from build123d import *

# Parameters (mm, degrees)
BOSS_EXTRUDE1_DEPTH = 15.7
LPATTERN1_COUNT     = 8
LPATTERN1_PITCH     = 8
SKETCH2_W           = 1.2
SKETCH2_H           = 6.1
CUT_EXTRUDE1_DEPTH  = 67.562602113
SKETCH3_W           = 0.8
SKETCH3_H           = 3.2
BOSS_EXTRUDE2_DEPTH = 15.7


with BuildPart() as part:
    # Sketch1 → Boss-Extrude1 (new body)
    with BuildSketch(Plane(origin=(0, 0, 0), x_dir=(1, 0, 0), z_dir=(0, 1, 0))):
        with BuildLine():
            Line((0, 10.8), (0, 15.5))
            Line((0, 15.5), (5.6, 15.5))
            Line((5.6, 15.5), (5.6, 10.8))
            Line((5.6, 10.8), (6.8, 10.8))
            Line((6.8, 10.8), (6.8, 9.75))
            ThreePointArc((6.8, 9.75), (4.8, 7.75), (6.8, 5.75))
            Line((6.8, 5.75), (6.8, 4.7))
            Line((6.8, 4.7), (5.6, 4.7))
            Line((5.6, 4.7), (5.6, 0))
            Line((5.6, 0), (0, 0))
            Line((0, 0), (0, 4.7))
            Line((0, 4.7), (-1.2, 4.7))
            Line((-1.2, 4.7), (-1.2, 5.75))
            ThreePointArc((-1.2, 5.75), (0.8, 7.75), (-1.2, 9.75))
            Line((-1.2, 9.75), (-1.2, 10.8))
            Line((-1.2, 10.8), (0, 10.8))
        make_face()
    boss_extrude1 = extrude(amount=BOSS_EXTRUDE1_DEPTH)

    # LPattern1: Boss-Extrude1 ×8
    with Locations(*[(i * LPATTERN1_PITCH, 0, 0) for i in range(1, LPATTERN1_COUNT)]):
        add(boss_extrude1)

    # Sketch2 → Cut-Extrude1 (cut, through all)
    with BuildSketch(Plane(origin=(0, 15.7, 0), x_dir=(1, 0, 0), z_dir=(0, 1, 0))):
        with Locations((-0.6, 7.75)):
            Rectangle(SKETCH2_W, SKETCH2_H)
        with Locations((62.2, 7.75)):
            Rectangle(SKETCH2_W, SKETCH2_H)
    extrude(amount=-CUT_EXTRUDE1_DEPTH, mode=Mode.SUBTRACT)

    # Sketch3 → Boss-Extrude2 (add)
    with BuildSketch(Plane(origin=(0, 15.7, 0), x_dir=(1, 0, 0), z_dir=(0, 1, 0))):
        with Locations((0.4, 7.75)):
            Rectangle(SKETCH3_W, SKETCH3_H)
        with Locations((61.2, 7.75)):
            Rectangle(SKETCH3_W, SKETCH3_H)
    extrude(amount=-BOSS_EXTRUDE2_DEPTH)


solid = part.part
Work out the finished part from the listing and answer in its coordinate system (mm). A direction names the side the tool comes from. Give positions to 0.01 mm unless a question says otherwise; leave off trailing zeros. Order: outer loops, then holes, each group sorted by start corner. A loop starts at its lowest first (then second) coordinate and runs counter-clockwise, first axis right, second up. Notation, with made-up numbers: (0, -35.5) -> (33, -35.5) arc R23 ccw to (33, -0.5) -> close; hole circle Ø7 at (65.5, 85.25). An arc over 180 degrees is marked (long way). Answer as a JSON object with one key per item and string values. Group by question number.
1. Flat-ended cylindrical pins translate along their axes: pin 1 Ø3.5 at (x, z) = (6.8, -7.75) entering from +Y; pin 2 Ø1.9 at (x, y) = (55, 5) entering from -Z. Find the tip coordinate at first contact, or state that the pin passes through.
2. Section A-A on x = 22.8 is taken. Determine the outline of the cut face in (y, z), plus the area to 3 significant figures.
3. A tool of negligible diameter and unlimited length cuts with its end or side. For faces 1 (the flat face through (47, 8, -10.8)), 2 (the flat face through (45.6, 8, -2)), 3 (the flat face through (51, 8, 0)), from which of +Z, -Z, +X, -X, +Y, -Y can it reach the whole face along a straight path? Write none if from no direction.
4. Consider line 1 along Z through (x, y) = (38.8, 11); line 2 along Z through (x, y) = (29.5, 14). Determine where each line is inside the solid, lowest interval first. Write a range as [from, to].
5. The mould has two halves that part along Z. Classify faces 4 (the flat face through (37.6, 8, -2)), 5 (the flat face through (23, 8, -4.7)), 6 (the flat face through (51, 8, -15.5)), 7 (the cylindrical face through (30.712, 7.74, -5.752)): released by +Z, released by -Z, zero draft, split by the parting line, or undercut.
6. Section B-B on z = -4 is taken. Count the separate pieces of the cut face and the enclosed holes in it, plus the area to 3 significant figures.
Result sheet:
{
 "1": {"pin 1": "passes through", "pin 2": "stops at z = -10.8"},
 "2": {"outline": "(0, -10.8) -> (15.7, -10.8) -> (15.7, -9.75) -> (0, -9.75) -> close; (0, -5.75) -> (15.7, -5.75) -> (15.7, -4.7) -> (0, -4.7) -> close", "area": "33.0 mm^2"},
 "3": {"face 1": "-Z, +Y, -Y", "face 2": "+Z, +Y, -Y", "face 3": "+Z, +X, -X, +Y, -Y"},
 "4": {"line 1": "z = [-10.8, -9.75], [-5.75, -4.7]", "line 2": "z = [-15.5, -9.27], [-6.23, 0]"},
 "5": {"face 4": "zero draft", "face 5": "released by +Z", "face 6": "released by -Z", "face 7": "undercut"},
 "6": {"separate pieces": "8", "enclosed holes": "0", "area": "703 mm^2"}
}
